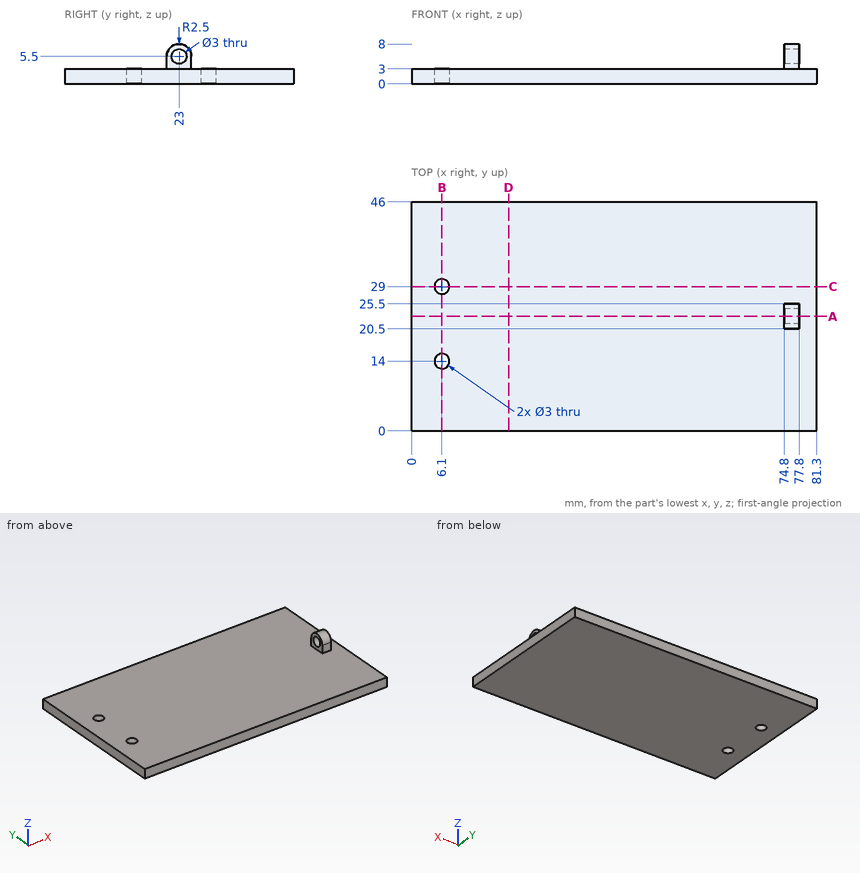
Job drawing, mm, ordinate dimensions from the low corner. One solid piece. Give positions to 0.01 mm unless a question says otherwise; leave off trailing zeros. Loops run counter-clockwise (first coordinate to the right, second up) from the corner with the lowest first, then second, coordinate; pieces in that order, holes last. Notation, with made-up numbers: (-7, 12) -> (46, 12) arc R24 cw to (46, 41) -> close; hole circle Ø3 at (-6, 80). An arc over 180 degrees is marked (long way). Write each question's results on one line, items separated by ' | '.
(1) Cut at B-B on x = 6.1. List the corners of the cut face in (y, z).
Geometry results:
outline: (0, 0) -> (12.5, 0) -> (12.5, 3) -> (0, 3) -> close; (15.5, 0) -> (27.5, 0) -> (27.5, 3) -> (15.5, 3) -> close; (30.5, 0) -> (46, 0) -> (46, 3) -> (30.5, 3) -> close
(2) Cut at D-D on x = 19.5. List the corners of the cut face in (y, z).
Geometry results:
outline: (0, 0) -> (46, 0) -> (46, 3) -> (0, 3) -> close
(3) Cut at C-C on y = 29. List the corners of the cut face in (x, z), and give its area (3 significant figures).
Geometry results:
outline: (0, 0) -> (4.6, 0) -> (4.6, 3) -> (0, 3) -> close; (7.6, 0) -> (81.3, 0) -> (81.3, 3) -> (7.6, 3) -> close | area: 235 mm²
(4) Flat gauge pins, fed straight in: pin 1 Ø1.8 at (y, z) = (23, 5.5) entering from -X; pin 2 Ø1.2 at (x, z) = (76.5, 4.5) entering from -Y; pin 3 Ø1.5 at (y, z) = (22, 5) entering from +X; pin 4 Ø14 at (x, y) = (59, 31.5) entering from +Z. Where does each tip first touch, or does it go through?
Geometry results:
pin 1: passes through | pin 2: stops at y = 20.5 | pin 3: stops at x = 77.8 | pin 4: stops at z = 3
(5) Cut at A-A on y = 23. List the corners of the cut face in (x, z), and give its area (3 significant figures).
Geometry results:
outline: (0, 0) -> (81.3, 0) -> (81.3, 3) -> (77.8, 3) -> (77.8, 4) -> (74.8, 4) -> (74.8, 3) -> (0, 3) -> close; (74.8, 7) -> (77.8, 7) -> (77.8, 8) -> (74.8, 8) -> close | area: 250 mm²
(6) Probe line 1 along Y through (x, z) = (6.1, 1.55); line 2 along Z through (x, y) = (29, 15); line 3 along Y through (x, z) = (77.1, 5.5). List the from-to ranges inside material, lowest first.
Geometry results:
line 1: y = 0 to 12.5, 15.5 to 27.5, 30.5 to 46 | line 2: z = 0 to 3 | line 3: y = 20.5 to 21.5, 24.5 to 25.5
